Check sheet for the modelled part. Datum: model origin and axes. Units: mm. A direction names the side the tool comes from. Round coordinates to 2 decimals unless told otherwise and drop trailing zeros. Loops run counter-clockwise (first coordinate to the right, second up) from the corner with the lowest first, then second, coordinate; pieces in that order, holes last. Notation, with made-up numbers: (-22.75, 27) -> (-11.75, 27) arc R26 cw to (-11.75, 64) -> close; hole circle Ø6 at (0, 69.5). An arc over 180 degrees is marked (long way). Return JSON: item names as keys, results as strings.
from build123d import *

# Parameters (mm, degrees)
MAIN_DEPTH                   = 35
SIDECUT_DEPTH                = 9.382441068
SIDECUT_DEPTH_BACK           = 21
SKETCH5_W                    = 45
SKETCH5_H                    = 60
CENTRALCUT_DEPTH             = 9.382441068
CENTRALCUT_DEPTH_BACK        = 21
SKETCH3_R                    = 1.6
MAKERBEAMFIXHOLES_DEPTH      = 1
MAKERBEAMFIXHOLES_DEPTH_BACK = 24.5
ROLLERSUPPORTHOLES_DEPTH     = 30
LPATTERN1_COUNT              = 3
LPATTERN1_PITCH              = 10
SKETCH6_R                    = 4.25
SCREWHOLE_DEPTH              = 3


with BuildPart() as part:
    # Sketch1 → Main (new body, symmetric)
    with BuildSketch(Plane.XY):
        Polygon((-10, 22.5), (-10, 18.842002095), (8.382441068, 0), (0, 0), (-20, 20.5), (-20, 22.5), (-16.45, 22.5), (-16.45, 23.5), (-13.55, 23.5), (-13.55, 22.5), align=None)
    extrude(amount=MAIN_DEPTH, both=True)

    # Sketch2 → SideCut (cut, two sides)
    with BuildSketch(Plane(origin=(0, 12.071067812, 0), x_dir=(0, 0, 1), z_dir=(1, 0, 0))) as sidecut_sk:
        Polygon((-35, -10.428932188), (-32.5, 12.071067812), (-35, 12.071067812), align=None)
        Polygon((35, -10.428932188), (35, 12.071067812), (32.5, 12.071067812), align=None)
    extrude(amount=SIDECUT_DEPTH, mode=Mode.SUBTRACT)
    extrude(sidecut_sk.sketch, amount=-SIDECUT_DEPTH_BACK, mode=Mode.SUBTRACT)

    # Sketch5 → CentralCut (cut, two sides)
    with BuildSketch(Plane(origin=(0, 0, 0), x_dir=(0, 0, 1), z_dir=(1, 0, 0))) as centralcut_sk:
        with Locations((0, 15.5)):
            Rectangle(SKETCH5_W, SKETCH5_H)
    extrude(amount=CENTRALCUT_DEPTH, mode=Mode.SUBTRACT)
    extrude(centralcut_sk.sketch, amount=-CENTRALCUT_DEPTH_BACK, mode=Mode.SUBTRACT)

    # Sketch3 → MakerBeamFixHoles (cut, two sides)
    with BuildSketch(Plane(origin=(0, 23.5, 0), x_dir=(1, 0, 0), z_dir=(0, 1, 0))) as makerbeamfixholes_sk:
        with Locations((-15, 15)):
            Circle(SKETCH3_R)
        with Locations((-15, -15)):
            Circle(SKETCH3_R)
    extrude(amount=MAKERBEAMFIXHOLES_DEPTH, mode=Mode.SUBTRACT)
    extrude(makerbeamfixholes_sk.sketch, amount=-MAKERBEAMFIXHOLES_DEPTH_BACK, mode=Mode.SUBTRACT)

    # Sketch4 → RollerSupportHoles (cut, symmetric)
    with BuildSketch(Plane.XY):
        with BuildLine():
            Line((-10.654722203, 10.921090258), (-8.559750647, 8.773744413))
            Line((-8.559750647, 8.773744413), (-7.486077724, 9.821230191))
            ThreePointArc((-7.486077724, 9.821230191), (-7.45989058, 11.942388892), (-9.58104928, 11.968576036))
            Line((-9.58104928, 11.968576036), (-10.654722203, 10.921090258))
        make_face()
    rollersupportholes = extrude(amount=ROLLERSUPPORTHOLES_DEPTH, both=True, mode=Mode.SUBTRACT)

    # LPattern1: RollerSupportHoles ×3
    with Locations(*[Vector(0.698323852, -0.715781948, 0) * (i * LPATTERN1_PITCH) for i in range(1, LPATTERN1_COUNT)]):
        add(rollersupportholes, mode=Mode.SUBTRACT)

    # Sketch6 → ScrewHole (cut)
    with BuildSketch(Plane(origin=(0, 14.5, 0), x_dir=(-1, 0, 0), z_dir=(0, -1, 0))):
        with Locations((15, 15)):
            Circle(SKETCH6_R)
        with Locations((15, -15)):
            Circle(SKETCH6_R)
    extrude(amount=-SCREWHOLE_DEPTH, mode=Mode.SUBTRACT)


solid = part.part
Q1. Section check B-B (z = 25). Record the boundary of the cut face in (x, y).
Results list:
{"outline": "(-20, 20.5) -> (-10.65, 10.92) -> (-9.58, 11.97) arc R1.5 cw to (-7.49, 9.82) -> (-8.56, 8.77) -> (-3.67, 3.76) -> (-2.6, 4.81) arc R1.5 cw to (-0.5, 2.66) -> (-1.58, 1.62) -> (0, 0) -> (8.38, 0) -> (-10, 18.84) -> (-10, 22.5) -> (-13.55, 22.5) -> (-13.55, 23.5) -> (-16.45, 23.5) -> (-16.45, 22.5) -> (-20, 22.5) -> close"}
Q2. Material ranges on line 1 (Z direction, x = -15, y = 18.95); line 2 (X direction, y = 21.25, z = 15); line 3 (Z direction, x = -15, y = 16.75), recorded low to high.
Results list:
{"line 1": "-34.61 to -16.6, -13.4 to 13.4, 16.6 to 34.61", "line 2": "-20 to -16.6, -13.4 to -10", "line 3": "-34.36 to -19.25, -10.75 to 10.75, 19.25 to 34.36"}
Q3. Section check A-A (z = 15). Record the boundary of the cut face in (x, y).
Results list:
{"outline": "(-20, 20.5) -> (-17.07, 17.5) -> (-16.6, 17.5) -> (-16.6, 22.5) -> (-20, 22.5) -> close; (-13.4, 17.5) -> (-10.75, 17.5) -> (-10.75, 14.5) -> (-5.76, 14.5) -> (-10, 18.84) -> (-10, 22.5) -> (-13.4, 22.5) -> close"}
Q4. Tool access check on faces 4 (the cylindrical face through (-7.44, 11.92, 26.3)), 5 (the flat face through (-10, 14.5, 0)), 6 (the flat face through (-18, 22.5, 0)), 7 (the flat face through (-13, 17.5, 15)). Record the directions out of +Z, -Z, +X, -X, +Y, -Y that give a thin tool (end or side, any length) a straight path to the whole face; none if there is none.
Results list:
{"face 4": "none", "face 5": "+X, -X, -Y", "face 6": "+Z, -Z, -X, +Y", "face 7": "-Y"}
Q5. Go/stop test with flat-tipped pins: pin 1 (3 mm diameter, centred on x = 2.5, z = 21.5, fed in from +Y); pin 2 (11.5 mm diameter, centred on x = -1, y = 8.5, fed in from +Z); pin 3 (11.5 mm diameter, centred on x = -4, y = 6.5, fed in from -Z); pin 4 (10 mm diameter, centred on x = -14, y = 5, fed in from -Z). Record where each tip stops, or that it passes through.
Results list:
{"pin 1": "y = 7.18", "pin 2": "z = 33.96", "pin 3": "z = -33.86", "pin 4": "through"}
Q6. Section check C-C (x = -15). Record the boundary of the cut face in (y, z) (3 decimals).
Results list:
{"outline": "(15.375, -34.208) -> (22.5, -35) -> (23.5, -35) -> (23.5, -16.6) -> (17.5, -16.6) -> (17.5, -19.25) -> (15.375, -19.25) -> close; (15.375, -10.75) -> (17.5, -10.75) -> (17.5, -13.4) -> (23.5, -13.4) -> (23.5, 13.4) -> (17.5, 13.4) -> (17.5, 10.75) -> (15.375, 10.75) -> close; (15.375, 19.25) -> (17.5, 19.25) -> (17.5, 16.6) -> (23.5, 16.6) -> (23.5, 35) -> (22.5, 35) -> (15.375, 34.208) -> close"}
Q7. Draft check along Y on faces 1 (the flat face through (-7.06, 15.83, 0.48)), 2 (the flat face through (-8, 11, -30)), 3 (the flat face through (-13, 17.5, -15)). Enter one of: released by +Y, released by -Y, zero draft, split by the parting line, or undercut.
Results list:
{"face 1": "released by +Y", "face 2": "undercut", "face 3": "released by -Y"}
Q8. Section check D-D (x = 6.5). Record the boundary of the cut face in (y, z), then the cut area to 3 significant figures.
Results list:
{"outline": "(0, -32.5) -> (1.93, -32.71) -> (1.93, -22.5) -> (0, -22.5) -> close; (0, 22.5) -> (1.93, 22.5) -> (1.93, 32.71) -> (0, 32.5) -> close", "area": "39.0 mm^2"}
